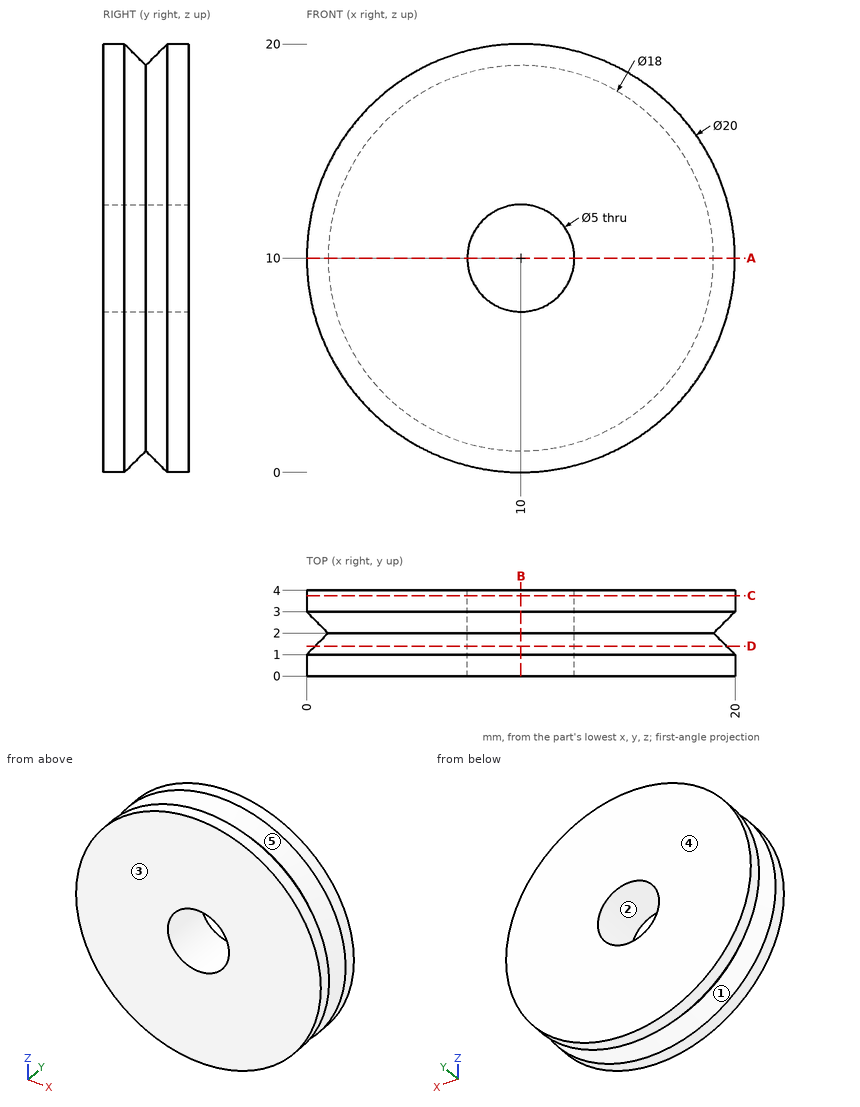
Could you check a few things on this drawing? It's one solid part, dimensions in mm from its lowest x, y, z. A direction names the side the tool comes from. Coordinates: 2 decimals unless noted, no trailing zeros. Order: outer loops, then holes, each group sorted by start corner. A loop starts at its lowest first (then second) coordinate and runs counter-clockwise, first axis right, second up. Notation, with made-up numbers: (24, -28) - (39, -28) arc R23 ccw to (39, -12) - close; hole circle Ø6 at (59.25, 22.25). An arc over 180 degrees is marked (long way). One line per question, with ' | ' between items.
(1) Suppose I cut it at D-D on y = 1.4. List the corners of the cut face in (x, z) for me, and give its area (3 significant figures).
Report:
outline: circle Ø19.2 at (10, 10); hole circle Ø5 at (10, 10) | area: 270 mm2
(2) Suppose I cut it at C-C on y = 3.75. List the corners of the cut face in (x, z) for me.
Report:
outline: circle Ø20 at (10, 10); hole circle Ø5 at (10, 10)
(3) Suppose I cut it at B-B on x = 10. List the corners of the cut face in (y, z) for me.
Report:
outline: (0, 0) - (1, 0) - (2, 1) - (3, 0) - (4, 0) - (4, 7.5) - (0, 7.5) - close; (0, 12.5) - (4, 12.5) - (4, 20) - (3, 20) - (2, 19) - (1, 20) - (0, 20) - close
(4) If we mould it in two halves opening along X, with no side actions, what happens to the marked faces 1, 2 and 3? For each: pulls with the +X half, pulls with the -X half, needs draft (parallel to the pull), parting line crosses it, or undercut.
Report:
face 1: parting line crosses it | face 2: undercut | face 3: needs draft
(5) Suppose I cut it at A-A on z = 10. List the corners of the cut face in (x, y) for me, and give its area (3 significant figures).
Report:
outline: (0, 0) - (7.5, 0) - (7.5, 4) - (0, 4) - (0, 3) - (1, 2) - (0, 1) - close; (12.5, 0) - (20, 0) - (20, 1) - (19, 2) - (20, 3) - (20, 4) - (12.5, 4) - close | area: 58.0 mm2
(6) If I drill on L1, parallel to Z at x = 10, y = 2.15; L2, parallel to Y at x = 5.75, z = 1.25; L3, parallel to Z at x = 10.75, y = 3.2, over which ranges is the centre line in solid material (lowest first)?
Report:
L1: z = 0.85 to 7.5, 12.5 to 19.15 | L2: y = 0 to 1.27, 2.73 to 4 | L3: z = 0.03 to 7.62, 12.38 to 19.97
(7) For the marked faces 4 and 5, which set-ups out of +Z, -Z, +X, -X, +Y, -Y let a thin tool reach every point of the face, with its end or its side?
Report:
face 4: +Z, -Z, +X, -X, +Y | face 5: none
(8) Will these pins go through, and if not, where does the flat tip stop? pin 1 (6.5 mm diameter, centred on x = 10, z = 10, fed in from -Y); pin 2 (1 mm diameter, centred on x = 18, y = 3, fed in from -Z).
Report:
pin 1: stops at y = 0 | pin 2: stops at z = 3.39
